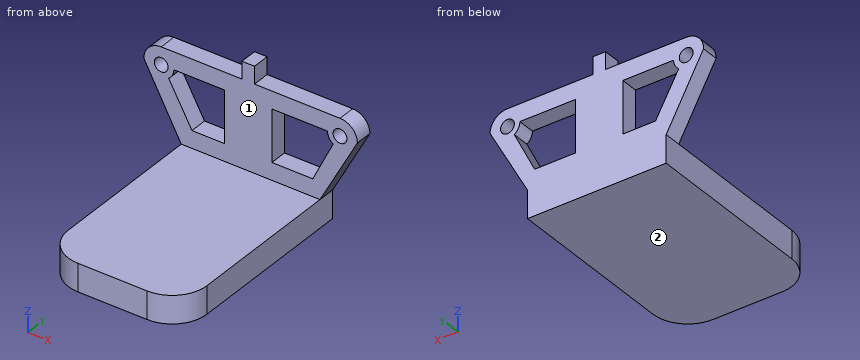
```python
from build123d import *

# Parameters (mm, degrees)
F0_W      = 40
F0_H      = 8
F1_DEPTH  = 60
F0_W_2    = 3.6288669872
F0_H_2    = 15
F0_R      = 2
F1_FACE_W = 40
F1_FACE_H = 8
F2_DEPTH  = 5
F3_R      = 10
F4_R      = 10
F5_DEPTH  = 25


with BuildPart() as f1:
    # F0 (on Front) → F1 (new body)
    with BuildSketch(Plane.XZ):
        with Locations((0, -4)):
            Rectangle(F0_W, F0_H)
    extrude(amount=F1_DEPTH)

    # F0 (on Front) + F1_face (on face) → F2 (join)
    with BuildSketch(Plane.XZ):
        with Locations((0, -4)):
            Rectangle(F0_W, F0_H)
        with BuildLine():
            Line((-30.7675590175, 19.8437826291), (-20, 0))
            Line((-20, 0), (20, 0))
            Line((20, 0), (30.77, 20))
            ThreePointArc((30.77, 20), (29.3055339059, 23.5355339059), (25.77, 25))
            Line((25.77, 25), (-25.77, 25))
            ThreePointArc((-25.77, 25), (-29.3603402941, 23.4798644475), (-30.7675590175, 19.8437826291))
        make_face()
        with BuildLine():
            ThreePointArc((-23.6389977535, 17.0627385142), (-22.5372148762, 18.3514321505), (-22.1411330128, 20))
            Line((-22.1411330128, 20), (-7.5, 20))
            Line((-7.5, 20), (-7.5, 5))
            Line((-7.5, 5), (-16.9122926891, 5))
            Line((-16.9122926891, 5), (-23.6389977535, 17.0627385142))
        make_face(mode=Mode.SUBTRACT)
        with Locations((-0.6855665064, 12.5)):
            Rectangle(F0_W_2, F0_H_2, mode=Mode.SUBTRACT)
        with Locations((-25.77, 20)):
            Circle(F0_R, mode=Mode.SUBTRACT)
        with BuildLine():
            Line((6.1288669872, 5), (6.1288669872, 20))
            Line((6.1288669872, 20), (22.1729351457, 20))
            ThreePointArc((22.1729351457, 20), (22.6057679037, 18.2892952308), (23.8001011411, 16.9902867159))
            Line((23.8001011411, 16.9902867159), (17.9096478969, 5))
            Line((17.9096478969, 5), (6.1288669872, 5))
        make_face(mode=Mode.SUBTRACT)
        with Locations((25.77, 20)):
            Circle(F0_R, mode=Mode.SUBTRACT)
    with BuildSketch(Plane(origin=(0, 0, -4), x_dir=(1, 0, 0), z_dir=(0, 1, 0))):
        Rectangle(F1_FACE_W, F1_FACE_H)
    extrude(amount=F2_DEPTH, dir=(0, -1, 0))

    # F3
    f3_edges = [f1.edges().sort_by_distance(p)[0] for p in [
        (-20, -60, -4),
    ]]
    fillet(f3_edges, radius=F3_R)

    # F4
    f4_edges = [f1.edges().sort_by_distance(p)[0] for p in [
        (20, -60, -4),
    ]]
    fillet(f4_edges, radius=F4_R)

    # F5 (add): a face of the model
    f5_faces = [f1.faces().sort_by_distance(p)[0] for p in [
        (-0.6855665064, -2.5, 5),
    ]]
    extrude(f5_faces, amount=F5_DEPTH)


solid = f1.part
```
For this review, take the finished solid that the model builds, in its own axes (mm). Face numbers are marked on the shaded views. A direction names the side the tool comes from. Coordinates: 2 decimals unless noted, no trailing zeros. Order: outer loops, then holes, each group sorted by start corner. A loop starts at its lowest first (then second) coordinate and runs counter-clockwise, first axis right, second up. Notation, with made-up numbers: (86.25, -13.5) -> (100.25, -13.5) arc R28 cw to (100.25, 16.5) -> close; hole circle Ø8 at (74, -32.5). An arc over 180 degrees is marked (long way). Use CSV: the item, a comma, the result in double quotes. Start each with the question number.
Item 1: For the marked faces 1 and 2, list the 3-axis set-ups (+Z, -Z, +X, -X, +Y, -Y) from which the entire face can be reached by the end or side of a thin tool; tool diameter is ignored.
Item 2: We need section A-A, the plane x = 13. Give the boundary of the cut face in (y, z).
Item 3: We need section C-C, the plane y = -39.5. Give the boundary of the cut face in (x, z).
Item 4: Wall thickness on probe 1 along X at (y, z) = (-3.5, -2); probe 2 along Y at (x, z) = (14.5, 1.5); probe 3 along Z at (x, y) = (-18, -16.5): over which ranges is each line inside the solid? List them lowest first.
Item 5: We need section D-D, the plane x = -19. Give the boundary of the cut face in (y, z), then the cut area to 3 significant figures.
Item 6: Insertion check: pin 1 (1.5 mm diameter, centred on x = 14.5, y = -3, fed in from +Z); pin 2 (1.5 mm diameter, centred on y = -3, z = 14.5, fed in from +X); pin 3 (12 mm diameter, centred on x = 8, y = -42.5, fed in from +Z). Each pin has a flat end and moves straight along its axis. Give the tip position at first contact, or say it passes through.
Item 7: We need section B-B, the plane z = 6. Give the boundary of the cut face in (x, y), then the cut area to 3 significant figures.
Derived:
1,face 1,"+Z, +X, -X, -Y"
1,face 2,"-Z, +X, -X, +Y, -Y"
2,outline,"(-59.54, -8) -> (0, -8) -> (0, 5) -> (-5, 5) -> (-5, 0) -> (-59.54, 0) -> close; (-5, 20) -> (0, 20) -> (0, 25) -> (-5, 25) -> close"
3,outline,"(-20, -8) -> (20, -8) -> (20, 0) -> (-20, 0) -> close"
4,probe 1,"x = -20 to 20"
4,probe 2,"y = -5 to 0"
4,probe 3,"z = -8 to 0"
5,outline,"(-54.36, -8) -> (0, -8) -> (0, 8.74) -> (-5, 8.74) -> (-5, 0) -> (-54.36, 0) -> close; (-5, 20) -> (0, 20) -> (0, 25) -> (-5, 25) -> close"
5,area,"504 mm^2"
6,pin 1,"stops at z = 25"
6,pin 2,"stops at x = 28.21"
6,pin 3,"stops at z = 0"
7,outline,"(-23.26, -5) -> (-17.47, -5) -> (-17.47, 0) -> (-23.26, 0) -> close; (-7.5, -5) -> (6.13, -5) -> (6.13, 0) -> (-7.5, 0) -> close; (18.4, -5) -> (23.23, -5) -> (23.23, 0) -> (18.4, 0) -> close"
7,area,"121 mm^2"
